Read the model definition and answer for the solid it produces. Units are mm, in the model's axes. A direction names the side the tool comes from. Round coordinates to 2 decimals unless told otherwise and drop trailing zeros. Loops run counter-clockwise (first coordinate to the right, second up) from the corner with the lowest first, then second, coordinate; pieces in that order, holes last. Notation, with made-up numbers: M 23.5,13 L 28.5,13 A23 ccw 28.5,40 Z; hole C 87.25,49 d8. An arc over 180 degrees is marked long. Write each question's results on one line, items separated by ' | '.
from build123d import *

# Parameters (mm, degrees)
BOSS_EXTRUDE1_DEPTH = 4
BOSS_EXTRUDE2_DEPTH = 8
BOSS_EXTRUDE3_DEPTH = 6


with BuildPart() as part:
    # Sketch1 → Boss-Extrude1 (new body)
    with BuildSketch(Plane(origin=(0, 0, 0), x_dir=(1, 0, 0), z_dir=(0, 1, 0))):
        with BuildLine():
            Line((31.75, -10), (31.75, 0))
            Line((31.75, 0), (24.25, 0))
            ThreePointArc((24.25, 0), (22.5, -1.75), (20.75, 0))
            Line((20.75, 0), (-20.75, 0))
            ThreePointArc((-20.75, 0), (-22.5, -1.75), (-24.25, 0))
            Line((-24.25, 0), (-31.75, 0))
            Line((-31.75, 0), (-31.75, -10))
            Line((-31.75, -10), (31.75, -10))
        make_face()
        with BuildLine():
            Line((24.25, 0), (31.75, 0))
            Line((31.75, 0), (31.75, 10))
            Line((31.75, 10), (-31.75, 10))
            Line((-31.75, 10), (-31.75, 0))
            Line((-31.75, 0), (-24.25, 0))
            ThreePointArc((-24.25, 0), (-22.5, 1.75), (-20.75, 0))
            Line((-20.75, 0), (20.75, 0))
            ThreePointArc((20.75, 0), (22.5, 1.75), (24.25, 0))
        make_face()
        with BuildLine():
            Line((31.75, -21.9), (31.75, -10))
            Line((31.75, -10), (-31.75, -10))
            Line((-31.75, -10), (-31.75, -21.9))
            ThreePointArc((-31.75, -21.9), (-29.275126266, -22.925126266), (-28.25, -25.4))
            Line((-28.25, -25.4), (28.25, -25.4))
            ThreePointArc((28.25, -25.4), (29.275126266, -22.925126266), (31.75, -21.9))
        make_face()
        with BuildLine():
            Line((-31.75, 10), (31.75, 10))
            Line((31.75, 10), (31.75, 21.9))
            ThreePointArc((31.75, 21.9), (29.275126266, 22.925126266), (28.25, 25.4))
            Line((28.25, 25.4), (-28.25, 25.4))
            ThreePointArc((-28.25, 25.4), (-29.275126266, 22.925126266), (-31.75, 21.9))
            Line((-31.75, 21.9), (-31.75, 10))
        make_face()
        with BuildLine():
            Line((36.195, -29.845), (36.195, -10))
            Line((36.195, -10), (31.75, -10))
            Line((31.75, -10), (31.75, -21.9))
            ThreePointArc((31.75, -21.9), (34.224873734, -22.925126266), (35.25, -25.4))
            ThreePointArc((35.25, -25.4), (31.75, -28.9), (28.25, -25.4))
            Line((28.25, -25.4), (-28.25, -25.4))
            ThreePointArc((-28.25, -25.4), (-34.224873734, -27.874873734), (-31.75, -21.9))
            Line((-31.75, -21.9), (-31.75, -10))
            Line((-31.75, -10), (-36.195, -10))
            Line((-36.195, -10), (-36.195, -29.845))
            Line((-36.195, -29.845), (36.195, -29.845))
        make_face()
        with BuildLine():
            Line((31.75, 10), (36.195, 10))
            Line((36.195, 10), (36.195, 29.845))
            Line((36.195, 29.845), (-36.195, 29.845))
            Line((-36.195, 29.845), (-36.195, 10))
            Line((-36.195, 10), (-31.75, 10))
            Line((-31.75, 10), (-31.75, 21.9))
            ThreePointArc((-31.75, 21.9), (-34.224873734, 27.874873734), (-28.25, 25.4))
            Line((-28.25, 25.4), (28.25, 25.4))
            ThreePointArc((28.25, 25.4), (31.75, 28.9), (35.25, 25.4))
            ThreePointArc((35.25, 25.4), (34.224873734, 22.925126266), (31.75, 21.9))
            Line((31.75, 21.9), (31.75, 10))
        make_face()
    extrude(amount=BOSS_EXTRUDE1_DEPTH)

    # Sketch1_3 → Boss-Extrude2 (add)
    with BuildSketch(Plane(origin=(0, 0, 0), x_dir=(1, 0, 0), z_dir=(0, 1, 0))):
        Polygon((39.75, -33.4), (39.75, -10), (36.195, -10), (36.195, -29.845), (-36.195, -29.845), (-36.195, -10), (-39.75, -10), (-39.75, -33.4), align=None)
        Polygon((36.195, 10), (39.75, 10), (39.75, 33.4), (-39.75, 33.4), (-39.75, 10), (-36.195, 10), (-36.195, 29.845), (36.195, 29.845), align=None)
    extrude(amount=BOSS_EXTRUDE2_DEPTH)

    # Sketch1_4 → Boss-Extrude3 (add)
    with BuildSketch(Plane(origin=(0, 0, 0), x_dir=(1, 0, 0), z_dir=(0, 1, 0))):
        with BuildLine():
            ThreePointArc((35.25, -25.4), (34.224873734, -22.925126266), (31.75, -21.9))
            Line((31.75, -21.9), (31.75, -23.65))
            ThreePointArc((31.75, -23.65), (32.987436867, -24.162563133), (33.5, -25.4))
            ThreePointArc((33.5, -25.4), (31.75, -27.15), (30, -25.4))
            Line((30, -25.4), (28.25, -25.4))
            ThreePointArc((28.25, -25.4), (31.75, -28.9), (35.25, -25.4))
        make_face()
        with BuildLine():
            Line((31.75, -23.65), (31.75, -21.9))
            ThreePointArc((31.75, -21.9), (29.275126266, -22.925126266), (28.25, -25.4))
            Line((28.25, -25.4), (30, -25.4))
            ThreePointArc((30, -25.4), (30.512563133, -24.162563133), (31.75, -23.65))
        make_face()
        with BuildLine():
            ThreePointArc((-28.25, -25.4), (-29.275126266, -22.925126266), (-31.75, -21.9))
            Line((-31.75, -21.9), (-31.75, -23.65))
            ThreePointArc((-31.75, -23.65), (-30.512563133, -24.162563133), (-30, -25.4))
            Line((-30, -25.4), (-28.25, -25.4))
        make_face()
        with BuildLine():
            Line((-31.75, -23.65), (-31.75, -21.9))
            ThreePointArc((-31.75, -21.9), (-34.224873734, -27.874873734), (-28.25, -25.4))
            Line((-28.25, -25.4), (-30, -25.4))
            ThreePointArc((-30, -25.4), (-32.987436867, -26.637436867), (-31.75, -23.65))
        make_face()
        with BuildLine():
            ThreePointArc((-28.25, 25.4), (-34.224873734, 27.874873734), (-31.75, 21.9))
            Line((-31.75, 21.9), (-31.75, 23.65))
            ThreePointArc((-31.75, 23.65), (-32.987436867, 26.637436867), (-30, 25.4))
            Line((-30, 25.4), (-28.25, 25.4))
        make_face()
        with BuildLine():
            Line((-31.75, 23.65), (-31.75, 21.9))
            ThreePointArc((-31.75, 21.9), (-29.275126266, 22.925126266), (-28.25, 25.4))
            Line((-28.25, 25.4), (-30, 25.4))
            ThreePointArc((-30, 25.4), (-30.512563133, 24.162563133), (-31.75, 23.65))
        make_face()
        with BuildLine():
            ThreePointArc((28.25, 25.4), (29.275126266, 22.925126266), (31.75, 21.9))
            Line((31.75, 21.9), (31.75, 23.65))
            ThreePointArc((31.75, 23.65), (30.512563133, 24.162563133), (30, 25.4))
            Line((30, 25.4), (28.25, 25.4))
        make_face()
        with BuildLine():
            Line((31.75, 23.65), (31.75, 21.9))
            ThreePointArc((31.75, 21.9), (34.224873734, 22.925126266), (35.25, 25.4))
            ThreePointArc((35.25, 25.4), (31.75, 28.9), (28.25, 25.4))
            Line((28.25, 25.4), (30, 25.4))
            ThreePointArc((30, 25.4), (31.75, 27.15), (33.5, 25.4))
            ThreePointArc((33.5, 25.4), (32.987436867, 24.162563133), (31.75, 23.65))
        make_face()
    extrude(amount=BOSS_EXTRUDE3_DEPTH)


solid = part.part
Item 1: The mould has two halves that part along Z. Classify faces 1 (the face through (36.195, 6, 20)), 2 (the face through (-1, 4, 33.4)), 3 (the face through (-39.75, 4, 22)): pulls with the +Z half, pulls with the -Z half, needs draft (parallel to the pull), parting line crosses it, or undercut.
Outcome:
face 1: undercut | face 2: pulls with the +Z half | face 3: needs draft
Item 2: The part is cut by section B-B (z = 0). Determine the outline of the cut face in (x, y).
Outcome:
outline: M -31.75,0 L -24.25,0 L -24.25,4 L -31.75,4 Z; M -20.75,0 L 20.75,0 L 20.75,4 L -20.75,4 Z; M 24.25,0 L 31.75,0 L 31.75,4 L 24.25,4 Z
Item 3: Flat-ended cylindrical pins translate along their axes: pin 1 (2 mm diameter, centred on x = -33, z = 27, fed in from +Y); pin 2 (3 mm diameter, centred on y = 2, z = 3, fed in from +X). Find the tip coordinate at first contact, or state that the pin passes through.
Outcome:
pin 1: stops at y = 6 | pin 2: stops at x = 31.75
Item 4: The part is cut by section C-C (x = -22.5). Determine the outline of the cut face in (y, z) (3 decimals), plus the area to 3 significant figures.
Outcome:
outline: M 0,-33.4 L 8,-33.4 L 8,-29.845 L 4,-29.845 L 4,-1.75 L 0,-1.75 Z; M 0,1.75 L 4,1.75 L 4,29.845 L 8,29.845 L 8,33.4 L 0,33.4 Z | area: 282 mm2
Item 5: The part is cut by section D-D (x = 9). Determine the outline of the cut face in (y, z) (3 decimals).
Outcome:
outline: M 0,-33.4 L 8,-33.4 L 8,-29.845 L 4,-29.845 L 4,29.845 L 8,29.845 L 8,33.4 L 0,33.4 Z
Item 6: For faces 4 (the face through (37, 3, 10)), 5 (the face through (-37, 3, 10)), 6 (the face through (-1, 6, -29.845)), determine the directions among +Z, -Z, +X, -X, +Y, -Y from which every point of the face is accessible in a straight line to the end or side of a thin tool.
Outcome:
face 4: +X, +Y, -Y | face 5: -X, +Y, -Y | face 6: +Y
Item 7: The part is cut by section A-A (y = 1). Determine the outline of the cut face in (x, z), plus the area to 3 significant figures.
Outcome:
outline: M -39.75,-33.4 L 39.75,-33.4 L 39.75,-10 L 31.75,-10 L 31.75,10 L 39.75,10 L 39.75,33.4 L -39.75,33.4 L -39.75,10 L -31.75,10 L -31.75,-10 L -39.75,-10 Z; hole C -31.75,-25.4 d3.5; hole C -31.75,25.4 d3.5; hole C -22.5,0 d3.5; hole C 22.5,0 d3.5; hole C 31.75,-25.4 d3.5; hole C 31.75,25.4 d3.5 | area: 4,930 mm2
Item 8: Straight lines are drawn through the part: line 1 (X direction, y = 2.55, z = 0); line 2 (X direction, y = 3.55, z = 25.4); line 3 (X direction, y = 6.5, z = 13.5) (3 decimals). For each, find the intervals that lie inside material, in ascending order.
Outcome:
line 1: x = -31.75 to -24.25, -20.75 to 20.75, 24.25 to 31.75 | line 2: x = -39.75 to -33.5, -30 to 30, 33.5 to 39.75 | line 3: x = -39.75 to -36.195, 36.195 to 39.75
